from build123d import *

# Parameters (mm, degrees)
SKETCH_R     = 12
PAD_DEPTH    = 37
SKETCH001_R  = 3.3
PAD001_DEPTH = 2
SKETCH002_R  = 6.5
PAD002_DEPTH = 3.8
SKETCH003_R  = 1.8
PAD003_DEPTH = 9


with BuildPart() as part:
    # Sketch → Pad (new body)
    with BuildSketch(Plane.YZ):
        Circle(SKETCH_R)
    extrude(amount=PAD_DEPTH)

    # Sketch001 (on Face3 of Pad) → Pad001 (join)
    with BuildSketch(Plane.YZ.offset(37)):
        Circle(SKETCH001_R)
    extrude(amount=PAD001_DEPTH)

    # Sketch002 (on Face2 of Pad001) → Pad002 (join)
    with BuildSketch(Plane(origin=(0, 0, 0), x_dir=(0, 1, 0), z_dir=(-1, 0, 0))):
        Circle(SKETCH002_R)
    extrude(amount=PAD002_DEPTH)

    # Sketch003 (on Face7 of Pad002) → Pad003 (join)
    with BuildSketch(Plane.YZ.offset(39)):
        Circle(SKETCH003_R)
    extrude(amount=PAD003_DEPTH)


solid = part.part
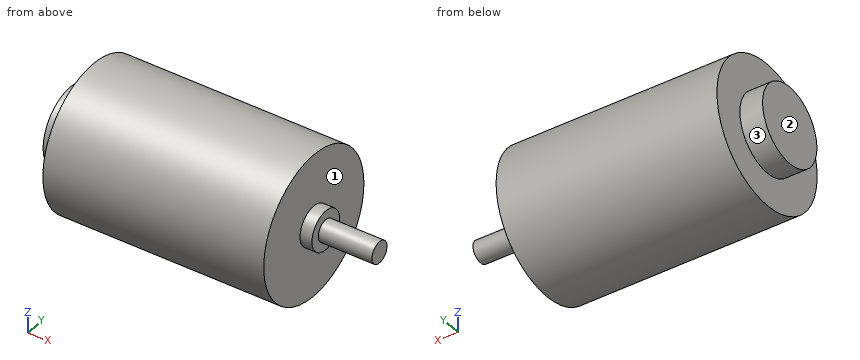
Geometry check sheet. Reference: the model listing, model coordinates, mm. Face numbers are marked on the shaded views. A direction names the side the tool comes from. Round coordinates to 2 decimals unless told otherwise and drop trailing zeros. Write each loop counter-clockwise with the first axis right and the second up, starting at its lowest first coordinate (ties: lowest second). Pieces come first, ordered by that corner, then holes.
Item 1: Section check C-C (x = 14.5). Record the boundary of the cut face in (y, z), plus the area to 3 significant figures.
Determined:
outline: circle Ø24 at (0, 0)
area: 452 mm2
Item 2: Section check D-D (y = -4.25). Record the boundary of the cut face in (x, z), plus the area to 3 significant figures.
Determined:
outline: (-3.8, -4.92) - (0, -4.92) - (0, -11.22) - (37, -11.22) - (37, 11.22) - (0, 11.22) - (0, 4.92) - (-3.8, 4.92) - close
area: 868 mm2
Item 3: Section check A-A (y = 0). Record the boundary of the cut face in (x, z).
Determined:
outline: (-3.8, -6.5) - (0, -6.5) - (0, -12) - (37, -12) - (37, -3.3) - (39, -3.3) - (39, -1.8) - (48, -1.8) - (48, 1.8) - (39, 1.8) - (39, 3.3) - (37, 3.3) - (37, 12) - (0, 12) - (0, 6.5) - (-3.8, 6.5) - close
Item 4: Go/stop test with flat-tipped pins: pin 1 Ø6 at (x, y) = (40.5, 2.5) entering from +Z; pin 2 Ø5 at (x, z) = (24, 5) entering from +Y; pin 3 Ø2 at (y, z) = (9, -2) entering from -X. Record where each tip stops, or that it passes through.
Determined:
pin 1: stops at z = 3.3
pin 2: stops at y = 11.74
pin 3: stops at x = 0
Item 5: Material ranges on line 1 along X through (y, z) = (-1.5, 9.25); line 2 along X through (y, z) = (3.75, -2); line 3 along Y through (x, z) = (4, 0.5), recorded low to high.
Determined:
line 1: x = 0 to 37
line 2: x = -3.8 to 37
line 3: y = -11.99 to 11.99
Item 6: Access from +Z, -Z, +X, -X, +Y, -Y to the whole of each face (thin tool, end or side, straight path). Record for the marked faces 1, 2 and 3.
Determined:
face 1: +X
face 2: +Z, -Z, -X, +Y, -Y
face 3: -X
